```python
from build123d import *

# Parameters (mm, degrees)
SKETCH2_W           = 0.8
SKETCH2_H           = 92
BOSS_EXTRUDE1_DEPTH = 8


with BuildPart() as part:
    # Sketch1 → Revolve1 (revolve)
    with BuildSketch(Plane(origin=(0, 0, 0), x_dir=(0, 0, -1), z_dir=(1, 0, 0))):
        Polygon((1.5, 0), (1.5, 8), (4, 8), (4, 12), (9, 12), (12, 8), (9, 4), (9, 0), align=None)
    revolve(axis=Axis((0, 55, 0), (0, -1, 0)))


with BuildPart() as body_2:
    # Mirror2: mirrored copy
    add(part.part.mirror(Plane.XY.offset(-50)))


with BuildPart() as part_1:
    add(part.part)

    add(body_2.part)  # Boss-Extrude1 merges body 2
    # Sketch2 → Boss-Extrude1 (add)
    with BuildSketch(Plane(origin=(0, 0, 0), x_dir=(1, 0, 0), z_dir=(0, 1, 0))):
        with Locations((0, 50)):
            Rectangle(SKETCH2_W, SKETCH2_H)
    extrude(amount=BOSS_EXTRUDE1_DEPTH)


solid = part_1.part
```
Read the model definition and answer for the solid it produces. Units are mm, in the model's axes. A direction names the side the tool comes from. Coordinates: 2 decimals unless noted, no trailing zeros. Loops run counter-clockwise (first coordinate to the right, second up) from the corner with the lowest first, then second, coordinate; pieces in that order, holes last. Notation, with made-up numbers: (85.25, -19) -> (110.25, -19) arc R36 ccw to (110.25, 20) -> close; hole circle Ø9 at (53.25, -7). An arc over 180 degrees is marked (long way). Return JSON: item names as keys, results as strings.
Item 1: For a pull along X with two mould halves and no side action, classify faces 1 (the conical face through (2.76, 11.75, -91.237)), 2 (the flat face through (-2, 8, -100)), 3 (the cylindrical face through (0.07, 4.06, 1.5)), 4 (the flat face through (-4, 12, 2)) as +X half, -X half, draft (parallel to the pull), parting line (faces both ways), or undercut.
Answers:
{"face 1": "parting line", "face 2": "undercut", "face 3": "undercut", "face 4": "draft"}
Item 2: Find section A-A (z = -100). Determine the outline of the cut face in (x, y).
Answers:
{"outline": "(-12, 8) -> (-9, 4) -> (-9, 0) -> (-1.5, 0) -> (-1.5, 8) -> (-4, 8) -> (-4, 12) -> (-9, 12) -> close; (1.5, 0) -> (9, 0) -> (9, 4) -> (12, 8) -> (9, 12) -> (4, 12) -> (4, 8) -> (1.5, 8) -> close"}
Item 3: For faces 5 (the flat face through (0, 0, -50)), 6 (the cylindrical face through (0, 10, -104)), 7 (the cylindrical face through (0, 2, 9)), determine the directions among +Z, -Z, +X, -X, +Y, -Y from which every point of the face is accessible in a straight line to the end or side of a thin tool.
Answers:
{"face 5": "+Z, -Z, +X, -X, -Y", "face 6": "+Y", "face 7": "-Y"}
Item 4: Find section C-C (z = -73). Determine the outline of the cut face in (x, y).
Answers:
{"outline": "(-0.4, 0) -> (0.4, 0) -> (0.4, 8) -> (-0.4, 8) -> close"}
Item 5: Flat-ended cylindrical pins translate along their axes: P1, Ø9, axis at x = 0, z = -100.5, coming from the +Y side; P2, Ø3.5, axis at x = 0, z = 0, coming from the +Y side; P3, Ø6.5, axis at y = 4, z = -63.5, coming from the +X side; P4, Ø8, axis at x = 8.5, z = -15.5, coming from the +Y side. Find the tip coordinate at first contact, or state that the pin passes through.
Answers:
{"P1": "stops at y = 12", "P2": "stops at y = 8", "P3": "stops at x = 0.4", "P4": "passes through"}
Item 6: Find the intervals of material crossed by probe 1 along Z at (x, y) = (-3.5, 11); probe 2 along X at (y, z) = (2.5, 0); probe 3 along Z at (x, y) = (-2, 9.5), in increasing order.
Answers:
{"probe 1": "z = -109.1 to -101.94, -98.06 to -90.9, -9.1 to -1.94, 1.94 to 9.1", "probe 2": "x = -9 to -1.5, 1.5 to 9", "probe 3": "z = -110.69 to -103.46, -96.54 to -89.31, -10.69 to -3.46, 3.46 to 10.69"}
Item 7: Find section B-B (y = 10.25). Determine the outline of the cut face in (x, z) (1 decimal).
Answers:
{"outline": "circle Ø20.6 at (0, -100); circle Ø20.6 at (0, 0); hole circle Ø8 at (0, -100); hole circle Ø8 at (0, 0)"}
